CAD build for the part. Positions are in the model's coordinates, mm. A direction names the side the tool comes from. Round coordinates to 2 decimals unless told otherwise and drop trailing zeros. Loops run counter-clockwise (first coordinate to the right, second up) from the corner with the lowest first, then second, coordinate; pieces in that order, holes last. Notation, with made-up numbers: (43.5, 32) -> (62.5, 32) arc R24 ccw to (62.5, 44) -> close; hole circle Ø2 at (76.25, 64.25). An arc over 180 degrees is marked (long way). Answer as CSV lines item,"result".
```python
from build123d import *

# Parameters (mm, degrees)
SKETCH1_R           = 4
BOSS_EXTRUDE2_DEPTH = 60
CHAMFER1_SIZE       = 0.2


with BuildPart() as part:
    # Sketch1 → Boss-Extrude2 (new body)
    with BuildSketch(Plane(origin=(0, 0, 0), x_dir=(1, 0, 0), z_dir=(0, 1, 0))):
        with Locations(Location((0, 0, 0), (0, 0, 270))):
            Circle(SKETCH1_R)
        Polygon((3.175, 0), (1.5875, 2.749630657), (-1.5875, 2.749630657), (-3.175, 0), (-1.5875, -2.749630657), (1.5875, -2.749630657), align=None, mode=Mode.SUBTRACT)
    extrude(amount=BOSS_EXTRUDE2_DEPTH)

    # Chamfer1
    chamfer1_edges = [part.edges().sort_by_distance(p)[0] for p in [
        (0, 0, -4),
        (0, 60, -4),
    ]]
    chamfer(chamfer1_edges, length=CHAMFER1_SIZE)


solid = part.part
```
Q1. Slice it at A-A, the plane x = 0. Give the cut face in (y, z).
Results:
outline,"(0, -3.8) -> (0.2, -4) -> (59.8, -4) -> (60, -3.8) -> (60, -2.75) -> (0, -2.75) -> close; (0, 2.75) -> (60, 2.75) -> (60, 3.8) -> (59.8, 4) -> (0.2, 4) -> (0, 3.8) -> close"
Q2. Two-plate mould, pull along Z, no slides. Class faces 1 (the flat face through (0, 30, 2.75)), 2 (the cylindrical face through (-3.905, 29.583, -0.867)), 3 (the flat face through (3, 0, -1)): pulls with the +Z half, pulls with the -Z half, needs draft (parallel to the pull), parting line crosses it, or undercut.
Results:
face 1,"undercut"
face 2,"parting line crosses it"
face 3,"needs draft"
Q3. Slice it at B-B, the plane y = 21. Give the cut face in (x, z) (1 decimal).
Results:
outline,"circle Ø8 at (0, 0); hole (-3.2, 0) -> (-1.6, -2.7) -> (1.6, -2.7) -> (3.2, 0) -> (1.6, 2.7) -> (-1.6, 2.7) -> close"
Q4. Tool access for faces 4 (the flat face through (2.37, 29.58, 1.394)), 5 (the flat face through (3, 60, -1)): list every direction of +Z, -Z, +X, -X, +Y, -Y with a clear straight run to the whole face (end or side of a thin tool).
Results:
face 4,"+Y, -Y"
face 5,"+Z, -Z, +X, -X, +Y"
Q5. Probe L1, parallel to Z at x = 1.25, y = 44.5; L2, parallel to Z at x = 0.25, y = 21; L3, parallel to X at y = 44, z = -1.5. List the from-to ranges inside material, lowest first. Write a range as [from, to].
Results:
L1,"[-3.8, -2.75], [2.75, 3.8]"
L2,"[-3.99, -2.75], [2.75, 3.99]"
L3,"[-3.71, -2.31], [2.31, 3.71]"
Q6. Drop flat-ended pins along their axis: pin 1 Ø3 at (y, z) = (30, -2) entering from -X; pin 2 Ø1 at (x, y) = (3, 47.5) entering from +Z; pin 3 Ø1 at (x, y) = (-0.5, 43.5) entering from -Z. Give the stop position or say it passes through.
Results:
pin 1,"x = -3.97"
pin 2,"z = 3.12"
pin 3,"z = -4"
